from build123d import *

# Parameters (mm, degrees)
CYLINDER019_R          = 1.6
CYLINDER019_DEPTH      = 23
ARRAY007_COUNT         = 4
CYLINDER016_R          = 4
CYLINDER016_DEPTH      = 350
CYLINDER018_R          = 5
CYLINDER018_DEPTH      = 10
CYLINDER017_R          = 11
CYLINDER017_DEPTH      = 2
CUT019_PLACEMENT_ANGLE = 45


with BuildPart() as array007:
    # Cylinder019 → Cylinder019 (new body)
    with BuildSketch(Plane(origin=(8, 0, 0), x_dir=(1, 0, 0), z_dir=(0, 0, 1))):
        Circle(CYLINDER019_R)
    extrude(amount=CYLINDER019_DEPTH)

    # Array007: Array007 ×4 about axis
    array007_axis = Axis((0, 0, 0), (0, 0, 1))


with BuildPart() as array007_1:
    add(array007.part)
    for i in range(1, ARRAY007_COUNT):
        add(array007.part.rotate(array007_axis, i * 360 / ARRAY007_COUNT))


with BuildPart() as cilindro016:
    # Cylinder016 → Cylinder016 (new body)
    with BuildSketch(Plane.XY):
        Circle(CYLINDER016_R)
    extrude(amount=CYLINDER016_DEPTH)


with BuildPart() as interior:
    # Cylinder018 → Cylinder018 (new body)
    with BuildSketch(Plane.XY):
        Circle(CYLINDER018_R)
    extrude(amount=CYLINDER018_DEPTH)


with BuildPart() as obj1:
    # Cylinder017 → Cylinder017 (new body)
    with BuildSketch(Plane.XY.offset(5)):
        Circle(CYLINDER017_R)
    extrude(amount=CYLINDER017_DEPTH)

    # Fusion018: union interior
    add(interior.part)


with BuildPart() as obj1_1:
    # Fusion018 placement: moved
    add(obj1.part.moved(Location((0, 0, 6))))

    # Cut018: cut Cilindro016
    add(cilindro016.part, mode=Mode.SUBTRACT)

    # Cut019: cut Array007
    add(array007_1.part, mode=Mode.SUBTRACT)


with BuildPart() as obj1_2:
    # Cut019 placement: moved
    add(obj1_1.part.moved(Location((22.5, -91, 22))).rotate(Axis((22.5, -91, 22), (0, 0, 1)), CUT019_PLACEMENT_ANGLE))


solid = obj1_2.part
Verification items for the finished model (mm, model axes). A direction names the side the tool comes from. Coordinates: 2 decimals unless noted, no trailing zeros. Write each loop counter-clockwise with the first axis right and the second up, starting at its lowest first coordinate (ties: lowest second). Pieces come first, ordered by that corner, then holes. Notation, with made-up numbers: (-36.5, 29.5) -> (14.5, 29.5) arc R20 ccw to (14.5, 34.5) -> close; hole circle Ø3 at (27.5, 53). An arc over 180 degrees is marked (long way). One line per item, written item: value. Start each with the question number.
Q1. Cross-section at B-B on x = 24.5. Enter the section's corners in (y, z).
Q2. Mould release check, pull along Y, two halves, no side actions. Record for faces 3 (the cylindrical face through (27.675, -98.183, 33.986)), 4 (the cylindrical face through (25.185, -95.218, 36.479)), 5 (the flat face through (27.5, -92.7, 35)): pulls with the +Y half, pulls with the -Y half, needs draft (parallel to the pull), parting line crosses it, or undercut.
Q3. Cross-section at A-A on y = -91. Enter the section's corners in (x, z), and give its area (3 significant figures).
Q4. Access from +Z, -Z, +X, -X, +Y, -Y to the whole of each face (thin tool, end or side, straight path). Record for faces 1 (the cylindrical face through (25.185, -95.218, 30.465)), 2 (the cylindrical face through (24.648, -94.374, 32.93)).
Q5. Cross-section at C-C on y = -86.5. Enter the section's corners in (x, z), and give its area (3 significant figures).
Q6. Thickness scan on L1, parallel to X at y = -91, z = 31; L2, parallel to Z at x = 30.75, y = -95.75; L3, parallel to X at y = -96.25, z = 34.75. Record the ranges inside material, lowest first. Write a range as from..to.
Q7. Go/stop test with flat-tipped pins: P1, Ø5, axis at x = 16.84, y = -96.66, coming from the -Z side; P2, Ø1, axis at x = 27.5, y = -94, coming from the +Z side; P3, Ø3, axis at x = 21, z = 29, coming from the -Y side; P4, Ø13, axis at x = 22.5, y = -91, coming from the -Z side. Record where each tip stops, or that it passes through.
Q8. Cross-section at D-D on z = 29. Enter the section's corners in (x, y).
Checked values:
1. outline: (-101.82, 33) -> (-95.58, 33) -> (-95.58, 28) -> (-94.46, 28) -> (-94.46, 38) -> (-95.58, 38) -> (-95.58, 35) -> (-101.82, 35) -> close; (-87.54, 28) -> (-86.42, 28) -> (-86.42, 33) -> (-80.18, 33) -> (-80.18, 35) -> (-86.42, 35) -> (-86.42, 38) -> (-87.54, 38) -> close
2. face 3: undercut
2. face 4: parting line crosses it
2. face 5: needs draft
3. outline: (11.5, 33) -> (17.5, 33) -> (17.5, 28) -> (18.5, 28) -> (18.5, 38) -> (17.5, 38) -> (17.5, 35) -> (11.5, 35) -> close; (26.5, 28) -> (27.5, 28) -> (27.5, 33) -> (33.5, 33) -> (33.5, 35) -> (27.5, 35) -> (27.5, 38) -> (26.5, 38) -> close
3. area: 44.0 mm²
4. face 1: -Z
4. face 2: +Z, -Z
5. outline: (12.46, 33) -> (15.74, 33) -> (15.74, 35) -> (12.46, 35) -> close; (17.95, 33) -> (20.32, 33) -> (20.32, 28) -> (24.68, 28) -> (24.68, 33) -> (27.05, 33) -> (27.05, 35) -> (24.68, 35) -> (24.68, 38) -> (20.32, 38) -> (20.32, 35) -> (17.95, 35) -> close; (29.26, 33) -> (32.54, 33) -> (32.54, 35) -> (29.26, 35) -> close
5. area: 66.2 mm²
6. L1: x = 17.5..18.5, 26.5..27.5
6. L2: z = 33..35
6. L3: x = 12.83..15.3, 18.39..26.61, 29.7..32.17
7. P1: stops at z = 33
7. P2: stops at z = 35
7. P3: stops at y = -96
7. P4: stops at z = 28
8. outline: circle Ø10 at (22.5, -91); hole circle Ø8 at (22.5, -91)
